from build123d import *

# Parameters (mm, degrees)
F0_R     = 2.032
F0_R_2   = 6.35
F1_DEPTH = 6.35


with BuildPart() as f1:
    # F0 (on Top) → F1 (new body)
    with BuildSketch(Plane.XY):
        with BuildLine():
            ThreePointArc((19.7957990072, -39.4337052755), (47.5560493208, -24.1519845894), (57.9235114877, 5.7926011118))
            ThreePointArc((57.9235114877, 5.7926011118), (56.3014842932, 16.7911237399), (51.5735114877, 26.8531685306))
            Line((51.5735114877, 26.8531685306), (51.5735114877, 37.5426011118))
            ThreePointArc((51.5735114877, 37.5426011118), (49.7136395482, 42.0327291723), (45.2235114877, 43.8926011118))
            Line((45.2235114877, 43.8926011118), (19.8235114877, 43.8926011118))
            Line((19.8235114877, 43.8926011118), (-5.5764885123, 43.8926011118))
            ThreePointArc((-5.5764885123, 43.8926011118), (-10.0666165728, 42.0327291723), (-11.9264885123, 37.5426011118))
            Line((-11.9264885123, 37.5426011118), (-11.9264885123, 26.8531685306))
            ThreePointArc((-11.9264885123, 26.8531685306), (-18.25813166, 6.9751640805), (-13.1720563965, -13.2573988882))
            Line((-13.1720563965, -13.2573988882), (-50.7122885123, -13.2573988882))
            Line((-50.7122885123, -13.2573988882), (-50.7122885123, -25.9573988882))
            Line((-50.7122885123, -25.9573988882), (-50.7122885123, -30.5437052755))
            ThreePointArc((-50.7122885123, -30.5437052755), (-48.1084677971, -36.8298845602), (-41.8222885123, -39.4337052755))
            Line((-41.8222885123, -39.4337052755), (19.7957990072, -39.4337052755))
        make_face()
        with Locations((-41.8222885123, -34.2946651749)):
            Circle(F0_R, mode=Mode.SUBTRACT)
        with BuildLine():
            ThreePointArc((17.7915114877, -34.2946651749), (19.8235114877, -32.2626651749), (21.8555114877, -34.2946651749))
            ThreePointArc((21.8555114877, -34.2946651749), (19.8235114877, -36.3266651749), (17.7915114877, -34.2946651749))
        make_face(mode=Mode.SUBTRACT)
        with Locations((-5.5764885123, 37.5426011118)):
            Circle(F0_R, mode=Mode.SUBTRACT)
        with Locations((19.8235114877, 5.7926011118)):
            Circle(F0_R_2, mode=Mode.SUBTRACT)
        with Locations((45.2235114877, 37.5426011118)):
            Circle(F0_R, mode=Mode.SUBTRACT)
    extrude(amount=F1_DEPTH)


solid = f1.part
Verification items for the finished model (mm, model axes). Give positions to 0.01 mm unless a question says otherwise; leave off trailing zeros. Order: outer loops, then holes, each group sorted by start corner. A loop starts at its lowest first (then second) coordinate and runs counter-clockwise, first axis right, second up. Notation, with made-up numbers: M 15.25,76 L 33.25,76 A36 ccw 33.25,113 Z; hole C 36.25,-12.75 d4. An arc over 180 degrees is marked long. Use one line per item in the form item = value. Start each with the question number.
Q1. Section check D-D (y = 31.5). Enter the section's corners in (x, z).
Q2. Section check A-A (y = 1). Enter the section's corners in (x, z), then the cut area to 3 significant figures.
Q3. Scan lines: line 1 along X through (y, z) = (-34.5, 3.5); line 2 along Y through (x, z) = (-20, 4); line 3 along X through (y, z) = (-35, 0.75). Record each from-to range of solid material in increasing order. Write a range as [from, to].
Q4. Section check B-B (x = -15). Enter the section's corners in (y, z).
Q5. Go/stop test with flat-tipped pins: pin 1 Ø4.5 at (x, y) = (19.82, -34.29) entering from +Z; pin 2 Ø2 at (y, z) = (-6, 1) entering from -X; pin 3 Ø1 at (x, z) = (-25.5, 3.5) entering from +Y. Record where each tip stops, or that it passes through.
Q6. Mould release check, pull along X, two halves, no side actions. Record for faces 1 (the cylindrical face through (47.26, -24.5, 3.13)), 2 (the cylindrical face through (47.162, 38.153, 3.131)), 3 (the flat face through (-11.926, 32, 3)), 4 (the flat face through (20, 43.893, 3)): +X half, -X half, draft (parallel to the pull), parting line (faces both ways), or undercut.
Q7. Section check C-C (z = 1.75). Enter the section's corners in (x, y).
Evaluation:
q1.outline = M -11.93,0 L 51.57,0 L 51.57,6.35 L -11.93,6.35 Z
q2.outline = M -17.97,0 L 15.66,0 L 15.66,6.35 L -17.97,6.35 Z; M 23.99,0 L 57.83,0 L 57.83,6.35 L 23.99,6.35 Z
q2.area = 428 mm2
q3.line_1 = [-49.78, -43.84], [-39.8, 17.8], [21.85, 34.86]
q3.line_2 = [-39.43, -13.26]
q3.line_3 = [-49.51, -43.73], [-39.92, 17.92], [21.73, 33.91]
q4.outline = M -39.43,0 L -13.26,0 L -13.26,6.35 L -39.43,6.35 Z; M -9.66,0 L 21.25,0 L 21.25,6.35 L -9.66,6.35 Z
q5.pin_1 = 6.35
q5.pin_2 = -16.72
q5.pin_3 = -13.26
q6.face_1 = +X half
q6.face_2 = undercut
q6.face_3 = -X half
q6.face_4 = draft
q7.outline = M -50.71,-30.54 A8.89 ccw -41.82,-39.43 L 19.8,-39.43 A44.14 ccw 57.92,5.79 A38.1 ccw 51.57,26.85 L 51.57,37.54 A6.35 ccw 45.22,43.89 L -5.58,43.89 A6.35 ccw -11.93,37.54 L -11.93,26.85 A38.1 ccw -13.17,-13.26 L -50.71,-13.26 Z; hole C -41.82,-34.29 d4.06; hole C -5.58,37.54 d4.06; hole C 19.82,5.79 d12.7; hole C 19.82,-34.29 d4.06; hole C 45.22,37.54 d4.06
